```python
from build123d import *

# Parameters (mm, degrees)
ESQUISSE1_W                      = 25
ESQUISSE1_H                      = 15
BOSS_EXTRU_1_DEPTH               = 37.2
BOSS_EXTRU_1_2_DEPTH             = 37.2
ESQUISSE3_W                      = 160
ESQUISSE3_H                      = 15
BOSS_EXTRU_2_DEPTH               = 15
ESQUISSE4_R                      = 5
ESQUISSE4_R_2                    = 4
BOSS_EXTRU_5_DEPTH               = 0.8
ESQUISSE4_6_R                    = 4
BOSS_EXTRU_6_DEPTH               = 7.4
CONG_1_R                         = 10
ESQUISSE5_W                      = 11
ESQUISSE5_H                      = 32.2
ENL_V_MAT_EXTRU_1_DEPTH          = 97.164442493
CONG_2_R                         = 10
ESQUISSE6_R                      = 1.75
ENL_V_MAT_EXTRU_2_DEPTH          = 100.613503101
ESQUISSE11_R                     = 1.75
TROUS_VIS_SUPPORT_CAPTEURS_DEPTH = 96.282999533
ESQUISSE12_W                     = 33.4
ESQUISSE12_H                     = 4.7
ENCOCHE_CARTE_CAPTEUR_DEPTH      = 96.282999533


with BuildPart() as part:
    # Esquisse1 → Boss.-Extru.1 (new body)
    with BuildSketch(Plane(origin=(0, 0, 0), x_dir=(0, 1, 0), z_dir=(0, 0, 1))):
        with Locations((-45, 0)):
            Rectangle(ESQUISSE1_W, ESQUISSE1_H)
    extrude(amount=BOSS_EXTRU_1_DEPTH)



with BuildPart() as body_2:
    # Esquisse1 → Boss.-Extru.1 2 (new body)
    with BuildSketch(Plane(origin=(0, 0, 0), x_dir=(0, 1, 0), z_dir=(0, 0, 1))):
        with Locations((45, 0)):
            Rectangle(ESQUISSE1_W, ESQUISSE1_H)
    extrude(amount=BOSS_EXTRU_1_2_DEPTH)


with BuildPart() as part_1:
    add(part.part)

    add(body_2.part)  # Boss.-Extru.2 merges body 2
    # Esquisse3 → Boss.-Extru.2 (add)
    with BuildSketch(Plane(origin=(0, 0, 0), x_dir=(0, 1, 0), z_dir=(0, 0, 1))):
        Rectangle(ESQUISSE3_W, ESQUISSE3_H)
    extrude(amount=-BOSS_EXTRU_2_DEPTH)

    # Esquisse4 → Boss.-Extru.5 (add)
    with BuildSketch(Plane(origin=(0, -80, 0), x_dir=(-1, 0, 0), z_dir=(0, -1, 0))):
        with Locations(Location((0, 7.5, 0), (0, 0, 90))):
            Circle(ESQUISSE4_R)
        with Locations(Location((0, 7.5, 0), (0, 0, 90))):
            Circle(ESQUISSE4_R_2, mode=Mode.SUBTRACT)
    boss_extru_5 = extrude(amount=BOSS_EXTRU_5_DEPTH)

    # Esquisse4<6> → Boss.-Extru.6 (add)
    with BuildSketch(Plane(origin=(0, -80, 0), x_dir=(-1, 0, 0), z_dir=(0, -1, 0))):
        with Locations(Location((0, 7.5, 0), (0, 0, 90))):
            Circle(ESQUISSE4_6_R)
    boss_extru_6 = extrude(amount=BOSS_EXTRU_6_DEPTH)

    # Symétrie2: Boss.-Extru.5, Boss.-Extru.6 across plane
    add(boss_extru_5.mirror(Plane.ZX))
    add(boss_extru_6.mirror(Plane.ZX))

    # Congé1
    cong_1_edges = [part_1.edges().sort_by_distance(p)[0] for p in [
        (0, 57.5, 0),
        (0, 32.5, 0),
        (0, -57.5, 0),
        (0, -32.5, 0),
    ]]
    fillet(cong_1_edges, radius=CONG_1_R)

    # Esquisse5 → Enlèv. mat.-Extru.1 (cut, through all)
    with BuildSketch(Plane(origin=(-7.5, 0, 0), x_dir=(0, -1, 0), z_dir=(-1, 0, 0))):
        with Locations((45, 16.1)):
            Rectangle(ESQUISSE5_W, ESQUISSE5_H)
        with Locations((-45, 16.1)):
            Rectangle(ESQUISSE5_W, ESQUISSE5_H)
    extrude(amount=-ENL_V_MAT_EXTRU_1_DEPTH, mode=Mode.SUBTRACT)

    # Congé2
    # the kernel refuses this fillet: 10 mm, written as the material it adds along each edge
    with BuildSketch(Plane(origin=(-7.5, 39.5, 0), x_dir=(0, 0, 1), z_dir=(1, 0, 0)), Plane(origin=(-7.5, -39.5, 0), x_dir=(0, -1, 0), z_dir=(1, 0, 0)), Plane(origin=(-7.5, -50.5, 0), x_dir=(0, 0, 1), z_dir=(1, 0, 0))) as cong_2_piece_1:
        with BuildLine():
            CenterArc((CONG_2_R, -CONG_2_R), CONG_2_R, 90, 90)
            Line((0, -CONG_2_R), (0, 0))
            Line((0, 0), (CONG_2_R, 0))
        make_face()
    extrude(amount=15)
    with BuildSketch(Plane(origin=(-7.5, 50.5, 0), x_dir=(0, 0, 1), z_dir=(1, 0, 0))) as cong_2_piece_2:
        with BuildLine():
            CenterArc((CONG_2_R, CONG_2_R), CONG_2_R, 180, 90)
            Line((0, CONG_2_R), (0, 0))
            Line((0, 0), (CONG_2_R, 0))
        make_face()
    extrude(amount=15)

    # Esquisse6 → Enlèv. mat.-Extru.2 (cut, through all)
    with BuildSketch(Plane(origin=(0, 0, 32.2), x_dir=(1, 0, 0), z_dir=(0, 0, -1))):
        with Locations(Location((0, 45, 0), (0, 0, 180))):
            Circle(ESQUISSE6_R)
        with Locations((0, -45)):
            Circle(ESQUISSE6_R)
    extrude(amount=-ENL_V_MAT_EXTRU_2_DEPTH, mode=Mode.SUBTRACT)

    # Esquisse11 → Trous vis support capteurs (cut, through all)
    with BuildSketch(Plane(origin=(0, 0, 0), x_dir=(0, 1, 0), z_dir=(0, 0, 1))):
        with Locations(Location((20, 0, 0), (0, 0, 270))):
            Circle(ESQUISSE11_R)
        with Locations(Location((-20, 0, 0), (0, 0, 270))):
            Circle(ESQUISSE11_R)
    extrude(amount=-TROUS_VIS_SUPPORT_CAPTEURS_DEPTH, mode=Mode.SUBTRACT)

    # Esquisse12 → Encoche carte capteur (cut, through all)
    with BuildSketch(Plane(origin=(0, 0, 0), x_dir=(0, 1, 0), z_dir=(0, 0, 1))):
        with Locations((-11.675958981, -8.388484641)):
            Rectangle(ESQUISSE12_W, ESQUISSE12_H)
    extrude(amount=-ENCOCHE_CARTE_CAPTEUR_DEPTH, mode=Mode.SUBTRACT)


solid = part_1.part
```
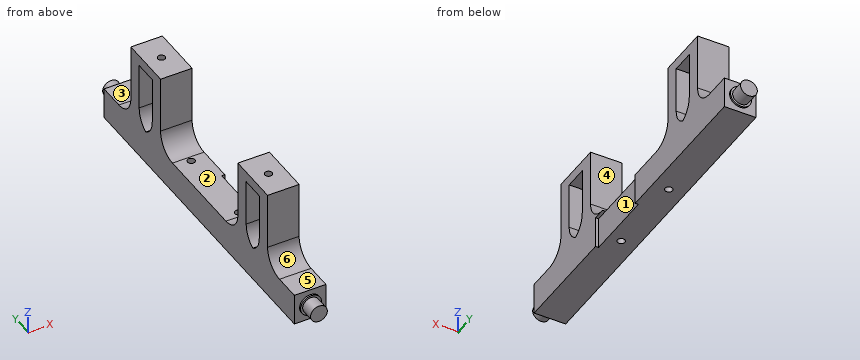
Work out the finished part from the listing and answer in its coordinate system (mm). Face numbers are marked on the shaded views. A direction names the side the tool comes from. Round coordinates to 2 decimals unless told otherwise and drop trailing zeros. Write each loop counter-clockwise with the first axis right and the second up, starting at its lowest first coordinate (ties: lowest second). Pieces come first, ordered by that corner, then holes. Notation, with made-up numbers: (10.25, 18.25) - (24.25, 18.25) arc R19 cw to (24.25, 33.25) - close; hole circle Ø9 at (-37.5, 12.25). An arc over 180 degrees is marked (long way). Return JSON: item names as keys, results as strings. Group by question number.
Q1. The part is cut by section C-C on z = -7.5. Write down the section's boundary in (x, y), then the cut area to 3 significant figures.
Q2. The part is cut by section D-D on y = 20. Write down the section's boundary in (x, z).
Q3. For the marked faces 1, 2 and 3, determine the directions among +Z, -Z, +X, -X, +Y, -Y from which every point of the face is accessible in a straight line to the end or side of a thin tool.
Q4. Find the intervals of material crossed by L1, parallel to Y at x = 0, z = -9.75; L2, parallel to Y at x = 6.25, z = 21.5; L3, parallel to Y at x = -1, z = -11.5, in increasing order.
Q5. The mould has two halves that part along Y. Classify the marked faces 4, 5 and 6: released by +Y, released by -Y, zero draft, split by the parting line, or undercut.
Q6. The part is cut by section A-A on y = -20. Write down the section's boundary in (x, z).
Q7. The part is cut by section B-B on z = 19.5. Write down the section's boundary in (x, y).
Q8. Each of these flat-tipped pins is pushed along its axis until it touches: pin 1 Ø2 at (x, z) = (-0.5, 22) entering from +Y; pin 2 Ø4.5 at (x, z) = (3.5, 26) entering from -Y; pin 3 Ø1.6 at (x, z) = (6.5, -8.5) entering from +Y; pin 4 Ø2 at (x, y) = (0, -20) entering from +Z. Where does it stop, or does it pass through?
Solved:
{
 "1": {"outline": "(-7.5, -80) - (-5, -80) - (-5, -80.8) - (-4, -80.8) - (-4, -87.4) - (4, -87.4) - (4, -80.8) - (5, -80.8) - (5, -80) - (7.5, -80) - (7.5, -28.38) - (6.04, -28.38) - (6.04, 5.02) - (7.5, 5.02) - (7.5, 80) - (5, 80) - (5, 80.8) - (4, 80.8) - (4, 87.4) - (-4, 87.4) - (-4, 80.8) - (-5, 80.8) - (-5, 80) - (-7.5, 80) - close; hole circle Ø3.5 at (0, -20); hole circle Ø3.5 at (0, 20)", "area": "2,450 mm²"},
 "2": {"outline": "(-7.5, -15) - (-1.75, -15) - (-1.75, 0) - (-7.5, 0) - close; (1.75, -15) - (7.5, -15) - (7.5, 0) - (1.75, 0) - close"},
 "3": {"face 1": "-Z, +X", "face 2": "+Z, +X, -X", "face 3": "+Z, +X, -X, +Y"},
 "4": {"L1": "-87.4 to -21.75, -18.25 to 18.25, 21.75 to 87.4", "L2": "-57.5 to -50.5, -39.5 to -32.5, 32.5 to 39.5, 50.5 to 57.5", "L3": "-80.8 to -21.44, -18.56 to 18.56, 21.44 to 80.8"},
 "5": {"face 4": "undercut", "face 5": "zero draft", "face 6": "released by -Y"},
 "6": {"outline": "(-7.5, -15) - (-1.75, -15) - (-1.75, 0) - (-7.5, 0) - close; (1.75, -15) - (6.04, -15) - (6.04, 0) - (1.75, 0) - close"},
 "7": {"outline": "(-7.5, -57.5) - (7.5, -57.5) - (7.5, -50.5) - (-7.5, -50.5) - close; (-7.5, -39.5) - (7.5, -39.5) - (7.5, -32.5) - (-7.5, -32.5) - close; (-7.5, 32.5) - (7.5, 32.5) - (7.5, 39.5) - (-7.5, 39.5) - close; (-7.5, 50.5) - (7.5, 50.5) - (7.5, 57.5) - (-7.5, 57.5) - close"},
 "8": {"pin 1": "y = 57.5", "pin 2": "y = -57.5", "pin 3": "y = 80", "pin 4": "through"}
}
